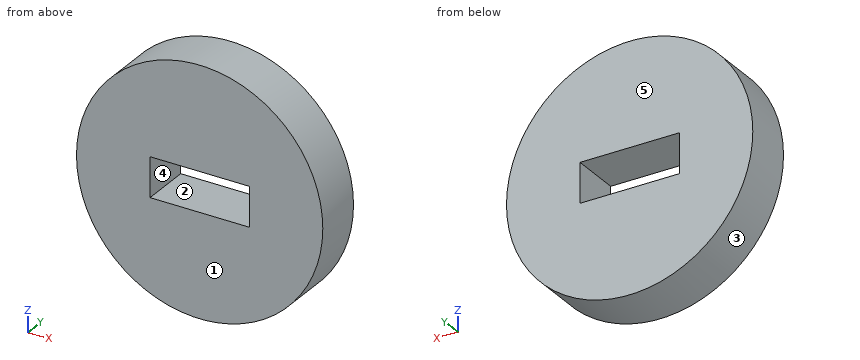
from build123d import *

# Parameters (mm, degrees)
F0_R     = 63.031777
F1_DEPTH = 12.7
F2_W     = 50.8
F2_H     = 20.32
F3_DEPTH = 25.401


with BuildPart() as f1:
    # F0 (on Front) → F1 (new body, symmetric)
    with BuildSketch(Plane.XZ):
        Circle(F0_R)
    extrude(amount=F1_DEPTH, both=True)

    # F2 (on face) → F3 (cut, through all)
    with BuildSketch(Plane.XZ.offset(12.7)):
        Rectangle(F2_W, F2_H)
    extrude(amount=-F3_DEPTH, mode=Mode.SUBTRACT)


solid = f1.part
Build history of the part. All positions in model axes, mm. Face numbers are marked on the shaded views. A direction names the side the tool comes from. Coordinates: 2 decimals unless noted, no trailing zeros. Order: outer loops, then holes, each group sorted by start corner. A loop starts at its lowest first (then second) coordinate and runs counter-clockwise, first axis right, second up. Notation, with made-up numbers: (86.25, 56.25) -> (115.25, 56.25) arc R35 cw to (115.25, 94.25) -> close; hole circle Ø7 at (79, 48). An arc over 180 degrees is marked (long way). One line per item, written item: value.
(1) Tool access for the marked faces 4 and 5: list every direction of +Z, -Z, +X, -X, +Y, -Y with a clear straight run to the whole face (end or side of a thin tool).
Checked values:
face 4: +Y, -Y
face 5: +Z, -Z, +X, -X, +Y
(2) Slice it at A-A, the plane z = 0. List the corners of the cut face in (x, y).
Checked values:
outline: (-63.03, -12.7) -> (-25.4, -12.7) -> (-25.4, 12.7) -> (-63.03, 12.7) -> close; (25.4, -12.7) -> (63.03, -12.7) -> (63.03, 12.7) -> (25.4, 12.7) -> close
(3) Slice it at C-C, the plane y = 0.5. List the corners of the cut face in (x, z), plus the area to 3 significant figures.
Checked values:
outline: circle Ø126.06 at (0, 0); hole (-25.4, -10.16) -> (25.4, -10.16) -> (25.4, 10.16) -> (-25.4, 10.16) -> close
area: 11,400 mm2
(4) Drop flat-ended pins along their axis: pin 1 Ø10 at (x, y) = (41.5, -7.5) entering from -Z; pin 2 Ø1.5 at (y, z) = (1, -40) entering from +X; pin 3 Ø1.5 at (x, y) = (24.5, 6.5) entering from +Z. Give the stop position or say it passes through.
Checked values:
pin 1: z = -51.39
pin 2: x = 49.32
pin 3: z = 58.39
(5) Slice it at D-D, the plane x = -27.5. List the corners of the cut face in (y, z).
Checked values:
outline: (-12.7, -56.72) -> (12.7, -56.72) -> (12.7, 56.72) -> (-12.7, 56.72) -> close
(6) Mould opens along X. For the marked faces 1, 2 and 3 say: pulls with the +X half, pulls with the -X half, needs draft (parallel to the pull), parting line crosses it, or undercut.
Checked values:
face 1: needs draft
face 2: undercut
face 3: parting line crosses it
(7) Slice it at B-B, the plane x = 0. List the corners of the cut face in (y, z), plus the area to 3 significant figures.
Checked values:
outline: (-12.7, -63.03) -> (12.7, -63.03) -> (12.7, -10.16) -> (-12.7, -10.16) -> close; (-12.7, 10.16) -> (12.7, 10.16) -> (12.7, 63.03) -> (-12.7, 63.03) -> close
area: 2,690 mm2
(8) Probe line 1 (X direction, y = 3.75, z = 9.5); line 2 (Z direction, x = 13, y = 10); line 3 (Z direction, x = 22.5, y = 0.75). List the from-to ranges inside material, lowest first. Write a range as [from, to].
Checked values:
line 1: [-62.31, -25.4], [25.4, 62.31]
line 2: [-61.68, -10.16], [10.16, 61.68]
line 3: [-58.88, -10.16], [10.16, 58.88]
